Read the model definition and answer for the solid it produces. Units are mm, in the model's axes. A direction names the side the tool comes from. Coordinates: 2 decimals unless noted, no trailing zeros. Write each loop counter-clockwise with the first axis right and the second up, starting at its lowest first coordinate (ties: lowest second). Pieces come first, ordered by that corner, then holes.
1) Which of the six approach directions +Z, -Z, +X, -X, +Y, -Y give full straight-line access (tool end or side, diameter ignored) to faces 1 (the face through (10, 74, 0)), 2 (the face through (50, 74, 30)), 3 (the face through (75, 74, 37))?
2) The part is cut by section D-D (x = -28). Determine the outline of the cut face in (y, z).
3) The part is cut by section B-B (z = 1). Determine the outline of the cut face in (x, y), then the cut area to 3 significant figures.
4) The part is cut by section A-A (x = 7.5). Determine the outline of the cut face in (y, z).
5) The part is cut by section C-C (y = 52.5). Determine the outline of the cut face in (x, z), then the cut area to 3 significant figures.
6) Each of these flat-tipped pins is pushed along its axis until it touches: pin 1 Ø22 at (y, z) = (48.5, 2.5) entering from +X; pin 2 Ø5 at (y, z) = (81, 26) entering from -X; pin 3 Ø8 at (x, y) = (59, 40.5) entering from -Z. Where does it stop, or does it pass through?
7) Determine the mould class of faces 4 (the face through (0, 74, 10)), 5 (the face through (-25, 74, 3)), 6 (the face through (-50, 74, 30)), 7 (the face through (25, 74, 2)) for opening direction X: +X half, -X half, draft (parallel to the pull), parting line (faces both ways), or undercut.
8) Find the intervals of material crossed by line 1 (X direction, y = 58.5, z = -3.5); line 2 (Z direction, x = 6.5, y = 99); line 3 (X direction, y = 10, z = -16), in increasing order.
from build123d import *

# Parameters (mm, degrees)
SKETCH1_W           = 20
SKETCH1_H           = 20
BOSS_EXTRUDE1_DEPTH = 150
CHAMFER1_SIZE       = 10


with BuildPart() as part:
    # Sketch1 → Boss-Extrude1 (new body)
    with BuildSketch(Plane(origin=(0, 0, 0), x_dir=(1, 0, 0), z_dir=(0, 1, 0))):
        Polygon((-25, 35), (25, 35), (25, -30), (75, -30), (75, -45), (-75, -45), (-75, -30), (-25, -30), align=None)
        Rectangle(SKETCH1_W, SKETCH1_H, mode=Mode.SUBTRACT)
    extrude(amount=BOSS_EXTRUDE1_DEPTH)

    # Chamfer1
    chamfer1_edges = [part.edges().sort_by_distance(p)[0] for p in [
        (-25, 75, -35),
        (25, 75, -35),
    ]]
    chamfer(chamfer1_edges, length=CHAMFER1_SIZE)


solid = part.part
Reported:
1. face 1: +Y, -Y
1. face 2: -Z, +X, +Y, -Y
1. face 3: +Z, -Z, +X, +Y, -Y
2. outline: (0, 30) - (150, 30) - (150, 45) - (0, 45) - close
3. outline: (-25, 0) - (-10, 0) - (-10, 150) - (-25, 150) - close; (10, 0) - (25, 0) - (25, 150) - (10, 150) - close
3. area: 4,500 mm2
4. outline: (0, -35) - (150, -35) - (150, -10) - (0, -10) - close; (0, 10) - (150, 10) - (150, 45) - (0, 45) - close
5. outline: (-75, 30) - (-25, 30) - (-25, -25) - (-15, -35) - (15, -35) - (25, -25) - (25, 30) - (75, 30) - (75, 45) - (-75, 45) - close; hole (-10, -10) - (10, -10) - (10, 10) - (-10, 10) - close
5. area: 5,000 mm2
6. pin 1: stops at x = 25
6. pin 2: stops at x = -25
6. pin 3: stops at z = 30
7. face 4: undercut
7. face 5: -X half
7. face 6: draft
7. face 7: +X half
8. line 1: x = -25 to -10, 10 to 25
8. line 2: z = -35 to -10, 10 to 45
8. line 3: x = -25 to 25
